The model under review builds one solid part; all positions refer to its coordinate system, in mm. A direction names the side the tool comes from. Coordinates: 2 decimals unless noted, no trailing zeros. Write each loop counter-clockwise with the first axis right and the second up, starting at its lowest first coordinate (ties: lowest second). Pieces come first, ordered by that corner, then holes. Notation, with made-up numbers: (-1.75, -23) -> (30.25, -23) arc R16 cw to (30.25, -7) -> close; hole circle Ø3 at (40.25, 66). An arc over 180 degrees is marked (long way). Put each result on its own line as item: value. Start each with the question number.
from build123d import *

# Parameters (mm, degrees)
F1_DEPTH = 1100
F3_DEPTH = 1100
F4_W     = 85.982085
F4_H     = 254.69566
F5_DEPTH = 25


with BuildPart() as f1:
    # F0 (on Front) → F1 (new body)
    with BuildSketch(Plane.XZ):
        Polygon((600, 150), (0, 150), (0, 0), (15, 0), (15, 135), (570, 135), (570, 0), (600, 0), align=None)
        Polygon((0, 0), (0, 150), (-600, 150), (-600, 0), (-570, 0), (-570, 135), (-15, 135), (-15, 0), align=None)
    extrude(amount=-F1_DEPTH)

    # F2 (on Front) → F3 (join)
    with BuildSketch(Plane.XZ):
        Polygon((0, -5), (0, 0), (-275.860757, 0), (-275.860757, 125.209585), (-479.573339, 125.209585), (-479.573339, 0), (-474.573339, 0), (-474.573339, 120.209585), (-280.860757, 120.209585), (-280.860757, -5), align=None)
        Polygon((474.573339, 0), (479.573339, 0), (479.573339, 125.209585), (275.860757, 125.209585), (275.860757, 0), (0, 0), (0, -5), (280.860757, -5), (280.860757, 120.209585), (474.573339, 120.209585), align=None)
    extrude(amount=-F3_DEPTH)

    # F4 (on face) → F5 (join)
    with BuildSketch(Plane(origin=(0, 0, 0), x_dir=(1, 0, 0), z_dir=(0, 0, -1))):
        with Locations((-583.983242, -144.877729)):
            Rectangle(F4_W, F4_H)
    extrude(amount=F5_DEPTH)


solid = f1.part
1. The part is to be moulded in two halves that separate along X. For faces 1 (the flat face through (600, 542, 74)), 2 (the flat face through (-614, 143, 0)), 3 (the flat face through (-275.861, 542, 62)), say which applies: released by +X, released by -X, zero draft, split by the parting line, or undercut.
2. Consider section C-C on y = 640.5. State the section outline as (x, z) points, then the cut area to 3 significant figures.
3. Tool access review of faces 4 (the flat face through (15, 542, 67)), 5 (the flat face through (-280.861, 542, 58)), 6 (the flat face through (-585, 17.53, -12)): name each direction out of +Z, -Z, +X, -X, +Y, -Y from which nothing blocks a thin tool from reaching the whole face with its end or side.
4. Consider section B-B on x = 163.5. State the section outline as (y, z) points.
5. Insertion check: P1, Ø21.5, axis at x = -615, y = 200, coming from the +Z side; P2, Ø20, axis at x = -576.5, z = -18, coming from the -Y side; P3, Ø3, axis at x = 269, y = 265, coming from the -Z side; P4, Ø20, axis at x = -591.5, z = -7, coming from the +Y side. Each pin has a flat end and moves straight along its axis. Give the tip position at first contact, or say it passes through.
6. Consider section A-A on z = 59. State the section outline as (x, y) points.
7. Wall thickness on line 1 (X direction, y = 835, z = 126); line 2 (Z direction, x = -419, y = 198); line 3 (Z direction, x = 163.5, y = 848.5): over which ranges is each line inside the solid? List them lowest first. Write a range as from..to.
Output values:
1. face 1: released by +X
1. face 2: zero draft
1. face 3: undercut
2. outline: (-600, 0) -> (-570, 0) -> (-570, 135) -> (-15, 135) -> (-15, 0) -> (-275.86, 0) -> (-275.86, 125.21) -> (-479.57, 125.21) -> (-479.57, 0) -> (-474.57, 0) -> (-474.57, 120.21) -> (-280.86, 120.21) -> (-280.86, -5) -> (280.86, -5) -> (280.86, 120.21) -> (474.57, 120.21) -> (474.57, 0) -> (479.57, 0) -> (479.57, 125.21) -> (275.86, 125.21) -> (275.86, 0) -> (15, 0) -> (15, 135) -> (570, 135) -> (570, 0) -> (600, 0) -> (600, 150) -> (-600, 150) -> close
2. area: 37,400 mm^2
3. face 4: +Y, -Y
3. face 5: -Z, +Y, -Y
3. face 6: -Z, -X, -Y
4. outline: (0, -5) -> (1100, -5) -> (1100, 0) -> (0, 0) -> close; (0, 135) -> (1100, 135) -> (1100, 150) -> (0, 150) -> close
5. P1: stops at z = 0
5. P2: stops at y = 17.53
5. P3: stops at z = -5
5. P4: stops at y = 1100
6. outline: (-600, 0) -> (-570, 0) -> (-570, 1100) -> (-600, 1100) -> close; (-479.57, 0) -> (-474.57, 0) -> (-474.57, 1100) -> (-479.57, 1100) -> close; (-280.86, 0) -> (-275.86, 0) -> (-275.86, 1100) -> (-280.86, 1100) -> close; (-15, 0) -> (15, 0) -> (15, 1100) -> (-15, 1100) -> close; (275.86, 0) -> (280.86, 0) -> (280.86, 1100) -> (275.86, 1100) -> close; (474.57, 0) -> (479.57, 0) -> (479.57, 1100) -> (474.57, 1100) -> close; (570, 0) -> (600, 0) -> (600, 1100) -> (570, 1100) -> close
7. line 1: x = -600..-570, -15..15, 570..600
7. line 2: z = 120.21..125.21, 135..150
7. line 3: z = -5..0, 135..150
